The listing builds one solid part. Answer for the finished solid, in the listing's coordinates (mm). Face numbers are marked on the shaded views. A direction names the side the tool comes from. Give positions to 0.01 mm unless a question says otherwise; leave off trailing zeros. Loops run counter-clockwise (first coordinate to the right, second up) from the corner with the lowest first, then second, coordinate; pieces in that order, holes last. Notation, with made-up numbers: M 33,51 L 84,51 A20 ccw 84,59 Z; hole C 15.25,57.5 d4. An arc over 180 degrees is marked long. Return JSON: item names as keys, results as strings.
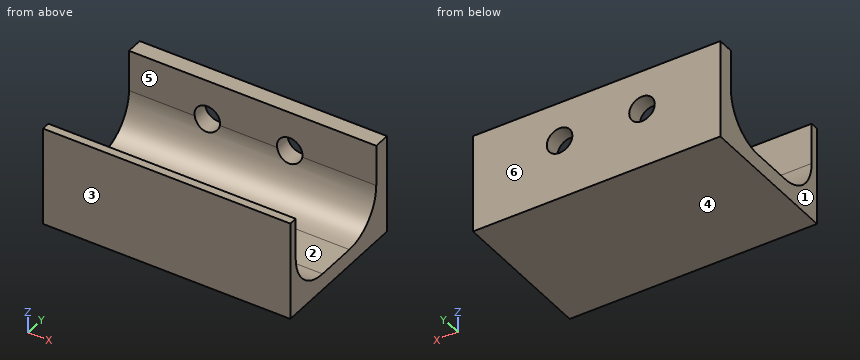
from build123d import *

# Parameters (mm, degrees)
BOSS_EXTRUDE1_DEPTH = 30
SKETCH2_R           = 1.55
CUT_EXTRUDE1_DEPTH  = 5


with BuildPart() as part:
    # Sketch1 → Boss-Extrude1 (new body)
    with BuildSketch(Plane(origin=(0, 0, 0), x_dir=(0, 0, -1), z_dir=(1, 0, 0))):
        with BuildLine():
            Line((-6.539148929, 14.609586507), (-11.539148929, 14.609586507))
            Line((-11.539148929, 14.609586507), (-11.539148929, 16.609586507))
            Line((-11.539148929, 16.609586507), (0.460851071, 16.609586507))
            Line((0.460851071, 16.609586507), (0.460851071, -1.390413493))
            Line((0.460851071, -1.390413493), (-11.539148929, -1.390413493))
            Line((-11.539148929, -1.390413493), (-11.539148929, -0.390413493))
            Line((-11.539148929, -0.390413493), (-8.539148929, -0.390413493))
            Line((-8.539148929, -0.390413493), (-6.539148929, -0.390413493))
            ThreePointArc((-6.539148929, -0.390413493), (-3.003615023, 1.074052601), (-1.539148929, 4.609586507))
            Line((-1.539148929, 4.609586507), (-1.539148929, 9.609586507))
            ThreePointArc((-1.539148929, 9.609586507), (-3.003615023, 13.145120413), (-6.539148929, 14.609586507))
        make_face()
    extrude(amount=BOSS_EXTRUDE1_DEPTH)

    # Sketch2 → Cut-Extrude1 (cut)
    with BuildSketch(Plane(origin=(0, 16.609586507, 0), x_dir=(1, 0, 0), z_dir=(0, 1, 0))):
        with Locations((-10.5, -6.789148929)):
            Circle(SKETCH2_R)
        with Locations((-20.5, -6.789148929)):
            Circle(SKETCH2_R)
        with Locations(Location((9.5, -6.789148929, 0), (0, 0, 270))):
            Circle(SKETCH2_R)
        with Locations(Location((19.5, -6.789148929, 0), (0, 0, 270))):
            Circle(SKETCH2_R)
    extrude(amount=-CUT_EXTRUDE1_DEPTH, mode=Mode.SUBTRACT)


solid = part.part
(1) Straight lines are drawn through the part: line 1 along Z through (x, y) = (19.5, 15.3); line 2 along Y through (x, z) = (15, 7.25); line 3 along Z through (x, y) = (18, 0). For each, find the intervals that lie inside material, in ascending order.
Values follow:
{"line 1": "-0.46 to 5.24, 8.34 to 11.54", "line 2": "-1.39 to -0.39, 14.61 to 16.61", "line 3": "-0.46 to 4.6"}
(2) Given pin 1 (5.5 mm diameter, centred on x = 8, y = 7, fed in from +Z), flat-ended and moving along its own axis, determine where the tip first touches the part or whether it passes through.
Values follow:
{"pin 1": "z = 1.55"}
(3) Determine the mould class of the marked faces 3, 4, 5 and 6 for opening direction Y: released by +Y, released by -Y, zero draft, split by the parting line, or undercut.
Values follow:
{"face 3": "released by -Y", "face 4": "zero draft", "face 5": "undercut", "face 6": "released by +Y"}
(4) The part is cut by section C-C (x = 5). Determine the outline of the cut face in (y, z), and give its area (3 significant figures).
Values follow:
{"outline": "M -1.39,-0.46 L 16.61,-0.46 L 16.61,11.54 L 14.61,11.54 L 14.61,6.54 A5 cw 9.61,1.54 L 4.61,1.54 A5 cw -0.39,6.54 L -0.39,11.54 L -1.39,11.54 Z", "area": "76.7 mm²"}
(5) The part is cut by section A-A (x = 19.5). Determine the outline of the cut face in (y, z).
Values follow:
{"outline": "M -1.39,-0.46 L 16.61,-0.46 L 16.61,5.24 L 14.44,5.24 A5 cw 9.61,1.54 L 4.61,1.54 A5 cw -0.39,6.54 L -0.39,11.54 L -1.39,11.54 Z; M 14.61,8.34 L 16.61,8.34 L 16.61,11.54 L 14.61,11.54 Z"}
(6) The part is cut by section B-B (z = 10.25). Determine the outline of the cut face in (x, y), and give its area (3 significant figures).
Values follow:
{"outline": "M 0,-1.39 L 30,-1.39 L 30,-0.39 L 0,-0.39 Z; M 0,14.61 L 30,14.61 L 30,16.61 L 0,16.61 Z", "area": "90.0 mm²"}
(7) The part is cut by section D-D (z = 8). Determine the outline of the cut face in (x, y).
Values follow:
{"outline": "M 0,-1.39 L 30,-1.39 L 30,-0.39 L 0,-0.39 Z; M 0,14.61 L 8.53,14.61 L 8.53,16.61 L 0,16.61 Z; M 10.47,14.61 L 18.53,14.61 L 18.53,16.61 L 10.47,16.61 Z; M 20.47,14.61 L 30,14.61 L 30,16.61 L 20.47,16.61 Z"}
(8) A tool of negligible diameter and unlimited length cuts with its end or side. For the marked faces 1 and 2, from which of +Z, -Z, +X, -X, +Y, -Y can it reach the whole face along a straight path? Write none if from no direction.
Values follow:
{"face 1": "+Z, -Z, -X, +Y, -Y", "face 2": "+Z, +X, -X"}
